from build123d import *

# Parameters (mm, degrees)
ESBO_O2_W                = 80
ESBO_O2_H                = 55
RESSALTO_EXTRUS_O1_DEPTH = 92
ESBO_O3_W                = 75
ESBO_O3_H                = 50
CORTE_EXTRUS_O1_DEPTH    = 89.5
ESBO_O4_W                = 35
ESBO_O4_H                = 15
CORTE_EXTRUS_O2_DEPTH    = 2.5
ESBO_O5_R                = 1
CORTE_EXTRUS_O3_DEPTH    = 125.980998556
ESBO_O6_W                = 10
ESBO_O6_H                = 10
RESSALTO_EXTRUS_O2_DEPTH = 2.5
ESBO_O8_R                = 1
CORTE_EXTRUS_O4_DEPTH    = 122.841085025


with BuildPart() as part:
    # Esboço2 → Ressalto-extrusão1 (new body)
    with BuildSketch(Plane(origin=(0, 0, 0), x_dir=(0, 0, -1), z_dir=(1, 0, 0))):
        Rectangle(ESBO_O2_W, ESBO_O2_H)
    extrude(amount=-RESSALTO_EXTRUS_O1_DEPTH)

    # Esboço3 → Corte-extrusão1 (cut)
    with BuildSketch(Plane(origin=(0, 0, 0), x_dir=(0, 0, -1), z_dir=(1, 0, 0))):
        Rectangle(ESBO_O3_W, ESBO_O3_H)
    extrude(amount=-CORTE_EXTRUS_O1_DEPTH, mode=Mode.SUBTRACT)

    # Esboço4 → Corte-extrusão2 (cut)
    with BuildSketch(Plane.ZY.offset(92)):
        with Locations((-20, 9)):
            Rectangle(ESBO_O4_W, ESBO_O4_H)
    extrude(amount=-CORTE_EXTRUS_O2_DEPTH, mode=Mode.SUBTRACT)

    # Esboço5 → Corte-extrusão3 (cut, through all)
    with BuildSketch(Plane.XY.offset(40)):
        with Locations((-9, 2.5)):
            Circle(ESBO_O5_R)
    extrude(amount=-CORTE_EXTRUS_O3_DEPTH, mode=Mode.SUBTRACT)

    # Esboço6 → Ressalto-extrusão2 (add)
    with BuildSketch(Plane(origin=(0, 0, 37.5), x_dir=(-1, 0, 0), z_dir=(0, 0, -1))):
        with Locations((9, 2.5)):
            Rectangle(ESBO_O6_W, ESBO_O6_H)
    ressalto_extrus_o2 = extrude(amount=RESSALTO_EXTRUS_O2_DEPTH)

    # Esboço8 → Corte-extrusão4 (cut, through all)
    with BuildSketch(Plane(origin=(0, 0, 35), x_dir=(-1, 0, 0), z_dir=(0, 0, -1))):
        with Locations(Location((9, 2.5, 0), (0, 0, 180))):
            Circle(ESBO_O8_R)
    corte_extrus_o4 = extrude(amount=-CORTE_EXTRUS_O4_DEPTH, mode=Mode.SUBTRACT)

    # Espelhar3: Ressalto-extrusão2, Corte-extrusão4 across plane
    add(ressalto_extrus_o2.mirror(Plane.XY))
    add(corte_extrus_o4.mirror(Plane.XY), mode=Mode.SUBTRACT)


solid = part.part
The model under review builds one solid part; all positions refer to its coordinate system, in mm. A direction names the side the tool comes from. Give positions to 0.01 mm unless a question says otherwise; leave off trailing zeros. Order: outer loops, then holes, each group sorted by start corner. A loop starts at its lowest first (then second) coordinate and runs counter-clockwise, first axis right, second up. Notation, with made-up numbers: M 27.5,-33 L 34.5,-33 A16 ccw 34.5,-18 Z; hole C 38.5,-23.75 d11. An arc over 180 degrees is marked long. One line per question, with ' | ' between items. Start each with the question number.
1) For faces 4 (the face through (-9, -2.5, -36)), 5 (the face through (-91, 9, -2.5)), 6 (the face through (-14, 2, -36)), list the 3-axis set-ups (+Z, -Z, +X, -X, +Y, -Y) from which the entire face can be reached by the end or side of a thin tool; tool diameter is ignored.
2) Consider section C-C, the plane x = -45. Give the boundary of the cut face in (y, z).
3) Clearance check with flat-ended pins moving along their axes: P1, Ø0.8, axis at y = 1.5, z = 37, coming from the +X side; P2, Ø6, axis at y = 17.5, z = -26.5, coming from the +X side; P3, Ø1.2, axis at y = 4.5, z = -36, coming from the -X side. State where each tip first meets the part, or that it passes through.
4) Consider section B-B, the plane z = -30.5. Give the boundary of the cut face in (x, y), then the cut area to 4 significant figures.
5) Consider section D-D, the plane z = 27. Give the boundary of the cut face in (x, y), then the cut area to 3 significant figures.
6) Consider section A-A, the plane y = 6. Give the boundary of the cut face in (x, z), then the cut area to 3 significant figures.
7) Wall thickness on L1, parallel to Y at x = -9, z = 36; L2, parallel to Y at x = -9, z = 38.95; L3, parallel to Z at x = -8.5, y = -14: over which ranges is each line inside the solid? List them lowest first. Write a range as from..to.
8) Mouldability with a two-part tool opening along Y and no side actions: class faces 1 (the face through (-44, 0, 37.5)), 2 (the face through (0, -26, 3)), 3 (the face through (-45, -27.5, 1)) as pulls with the +Y half, pulls with the -Y half, needs draft (parallel to the pull), parting line crosses it, or undercut.
Found:
1) face 4: +X | face 5: +X, -X | face 6: none
2) outline: M -27.5,-40 L 27.5,-40 L 27.5,40 L -27.5,40 Z; hole M -25,-37.5 L 25,-37.5 L 25,37.5 L -25,37.5 Z
3) P1: stops at x = -4 | P2: stops at x = -89.5 | P3: stops at x = -14
4) outline: M -92,-27.5 L 0,-27.5 L 0,-25 L -89.5,-25 L -89.5,1.5 L -92,1.5 Z; M -92,16.5 L -89.5,16.5 L -89.5,25 L 0,25 L 0,27.5 L -92,27.5 Z | area: 547.5 mm²
5) outline: M -92,-27.5 L 0,-27.5 L 0,-25 L -89.5,-25 L -89.5,25 L 0,25 L 0,27.5 L -92,27.5 Z | area: 585 mm²
6) outline: M -92,-40 L 0,-40 L 0,-37.5 L -4,-37.5 L -4,-35 L -14,-35 L -14,-37.5 L -92,-37.5 Z; M -92,-2.5 L -89.5,-2.5 L -89.5,37.5 L -14,37.5 L -14,35 L -4,35 L -4,37.5 L 0,37.5 L 0,40 L -92,40 Z | area: 610 mm²
7) L1: y = -27.5..-25, -2.5..1.5, 3.5..7.5, 25..27.5 | L2: y = -27.5..1.5, 3.5..27.5 | L3: z = -40..-37.5, 37.5..40
8) face 1: undercut | face 2: needs draft | face 3: pulls with the -Y half
